CAD build for the part. Positions are in the model's coordinates, mm. Face numbers are marked on the shaded views. A direction names the side the tool comes from. Coordinates: 2 decimals unless noted, no trailing zeros. Write each loop counter-clockwise with the first axis right and the second up, starting at its lowest first coordinate (ties: lowest second). Pieces come first, ordered by that corner, then holes. Notation, with made-up numbers: M 22.5,89.25 L 51.5,89.25 A22 ccw 51.5,105.25 Z; hole C 56,-33.5 d10. An arc over 180 degrees is marked long. Put each result on its own line as item: value. Start each with the question number.
```python
from build123d import *

# Parameters (mm, degrees)
F0_R     = 12.4968
F1_DEPTH = 11.1252
F2_DEPTH = 6.35


with BuildPart() as f1:
    # F0 (on Front) → F1 (new body)
    with BuildSketch(Plane.XZ):
        Circle(F0_R)
        with BuildLine():
            ThreePointArc((7.394862, 3.668929), (8.037089, 1.884202), (8.255, 0))
            ThreePointArc((8.255, 0), (8.254842, -0.051077), (8.254368, -0.102152))
            ThreePointArc((8.254368, -0.102152), (10.104053, -0.374671), (10.95885, -2.037478))
            ThreePointArc((10.95885, -2.037478), (9.703631, -3.923616), (7.479105, -3.493997))
            ThreePointArc((7.479105, -3.493997), (6.452437, -5.148891), (5.066648, -6.517216))
            ThreePointArc((5.066648, -6.517216), (5.758448, -7.257852), (6.009617, -8.23971))
            ThreePointArc((6.009617, -8.23971), (3.85785, -10.281605), (1.931429, -8.025871))
            ThreePointArc((1.931429, -8.025871), (-0.002536, -8.255), (-1.936361, -8.024683))
            ThreePointArc((-1.936361, -8.024683), (-1.928052, -8.130833), (-1.925279, -8.237272))
            ThreePointArc((-1.925279, -8.237272), (-4.952388, -10.030501), (-5.070652, -6.514101))
            ThreePointArc((-5.070652, -6.514101), (-6.4556, -5.144925), (-7.481251, -3.4894))
            ThreePointArc((-7.481251, -3.4894), (-10.847828, -2.70022), (-8.687861, 0))
            Line((-8.687861, 0), (-8.255, 0))
            ThreePointArc((-8.255, 0), (-8.03651, 1.886672), (-7.392606, 3.673472))
            ThreePointArc((-7.392606, 3.673472), (-8.745562, 6.97875), (-5.222453, 6.393044))
            ThreePointArc((-5.222453, 6.393044), (-3.579425, 7.438598), (-1.737178, 8.070145))
            ThreePointArc((-1.737178, 8.070145), (-0.555332, 11.111082), (2.04751, 9.144035))
            ThreePointArc((2.04751, 9.144035), (1.969685, 8.585289), (1.742137, 8.069076))
            ThreePointArc((1.742137, 8.069076), (3.583995, 7.436397), (5.22638, 6.389834))
            ThreePointArc((5.22638, 6.389834), (7.501448, 7.713433), (9.195546, 5.699016))
            ThreePointArc((9.195546, 5.699016), (8.680509, 4.342207), (7.394862, 3.668929))
        make_face(mode=Mode.SUBTRACT)
    extrude(amount=F1_DEPTH)

    # F0 (on Front) → F2 (join)
    with BuildSketch(Plane.XZ):
        with BuildLine():
            ThreePointArc((8.254368, -0.102152), (8.254842, -0.051077), (8.255, 0))
            ThreePointArc((8.255, 0), (8.037089, 1.884202), (7.394862, 3.668929))
            ThreePointArc((7.394862, 3.668929), (5.551844, 4.424657), (5.22638, 6.389834))
            ThreePointArc((5.22638, 6.389834), (3.583995, 7.436397), (1.742137, 8.069076))
            ThreePointArc((1.742137, 8.069076), (0.002181, 7.099335), (-1.737178, 8.070145))
            ThreePointArc((-1.737178, 8.070145), (-3.579425, 7.438598), (-5.222453, 6.393044))
            ThreePointArc((-5.222453, 6.393044), (-5.132818, 6.053392), (-5.102643, 5.703409))
            ThreePointArc((-5.102643, 5.703409), (-5.791004, 4.173329), (-7.392606, 3.673472))
            ThreePointArc((-7.392606, 3.673472), (-8.03651, 1.886672), (-8.255, 0))
            Line((-8.255, 0), (0, 0))
            Line((0, 0), (0, -2.032))
            Line((0, -2.032), (-6.8707, -2.032))
            ThreePointArc((-6.8707, -2.032), (-7.029505, -2.822061), (-7.481251, -3.4894))
            ThreePointArc((-7.481251, -3.4894), (-6.4556, -5.144925), (-5.070652, -6.514101))
            ThreePointArc((-5.070652, -6.514101), (-3.082251, -6.395333), (-1.936361, -8.024683))
            ThreePointArc((-1.936361, -8.024683), (-0.002536, -8.255), (1.931429, -8.025871))
            ThreePointArc((1.931429, -8.025871), (3.078321, -6.397226), (5.066648, -6.517216))
            ThreePointArc((5.066648, -6.517216), (6.452437, -5.148891), (7.479105, -3.493997))
            ThreePointArc((7.479105, -3.493997), (6.920854, -1.581877), (8.254368, -0.102152))
        make_face()
        with BuildLine():
            Line((0, 0), (-8.255, 0))
            ThreePointArc((-8.255, 0), (-8.254857, -0.048541), (-8.254429, -0.09708))
            ThreePointArc((-8.254429, -0.09708), (-7.252228, -0.842607), (-6.8707, -2.032))
            Line((-6.8707, -2.032), (0, -2.032))
            Line((0, -2.032), (0, 0))
        make_face()
    extrude(amount=F2_DEPTH)


solid = f1.part
```
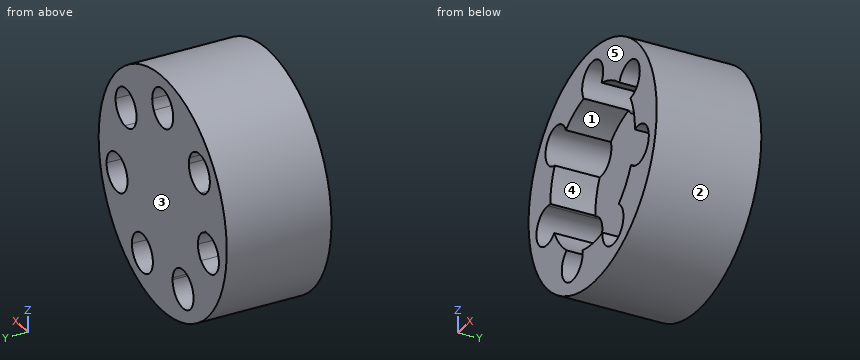
(1) Drill centre lines: line 1 (X direction, y = -10, z = -10); line 2 (X direction, y = -4.25, z = -9.25); line 3 (X direction, y = -2, z = 7.5). Where is each one in solid material? Low to high. Write a range as [from, to].
(2) Slice it at D-D, the plane z = 6.75. Write the cut outline in (x, y), then the cut area to 3 significant figures.
(3) Slice it at A-A, the plane x = 0. Write the cut outline in (y, z) (3 decimals), then the cut area to 3 significant figures.
(4) Which spindle directions (+Z, -Z, +X, -X, +Y, -Y) get a long thin tool onto all of the face, cutting with end or side? Do the marked faces 4 and 5. Say none if no direction does.
(5) Two-plate mould, pull along Z, no slides. Class the marked faces 1, 2 and 3: +Z half, -Z half, draft (parallel to the pull), parting line (faces both ways), or undercut.
(6) Slice it at B-B, the plane y = -2. State how many separate pieces and enclosed holes the cut face has, then the cut area to 3 significant figures.
(7) Drop flat-ended pins along their axis: pin 1 (1 mm diameter, centred on x = 6, y = -10, fed in from +Z); pin 2 (2 mm diameter, centred on y = -7, z = -3, fed in from -X); pin 3 (3.5 mm diameter, centred on x = -3.97, z = -8.24, fed in from +Y); pin 4 (2 mm diameter, centred on y = -1.5, z = -4, fed in from -X). Give the stop position or say it passes through.
Result set:
1. line 1: x = [-7.49, -5.01], [-2.93, 2.92], [5.01, 7.49]
1. line 2: x = [-8.4, -5.75], [-2.19, 2.19], [5.74, 8.4]
1. line 3: x = [-10, -8.12], [-6.17, -1.21], [1.22, 6.18], [8.12, 10]
2. outline: M -10.52,-11.13 L -8.9,-11.13 L -8.9,0 L -10.52,0 Z; M -5.39,-11.13 L -4.75,-11.13 L -4.75,-6.35 L 4.75,-6.35 L 4.75,-11.13 L 5.4,-11.13 L 5.4,0 L -5.39,0 Z; M 8.9,-11.13 L 10.52,-11.13 L 10.52,0 L 8.9,0 Z
2. area: 111 mm^2
3. outline: M -11.125,-12.497 L 0,-12.497 L 0,7.099 L -6.35,7.099 L -6.35,-8.255 L -11.125,-8.255 Z; M -11.125,11.189 L 0,11.189 L 0,12.497 L -11.125,12.497 Z
3. area: 159 mm^2
4. face 4: -Y
4. face 5: +Z, -Z, +X, -X, -Y
5. face 1: undercut
5. face 2: parting line
5. face 3: draft
6. separate pieces: 1
6. enclosed holes: 7
6. area: 399 mm^2
7. pin 1: stops at z = 11.22
7. pin 2: stops at x = -12.34
7. pin 3: passes through
7. pin 4: stops at x = -12.13
